Geometry: final body of the model. Coordinates: model frame, mm. A direction names the side the tool comes from. Coordinates: 2 decimals unless noted, no trailing zeros. Write each loop counter-clockwise with the first axis right and the second up, starting at its lowest first coordinate (ties: lowest second). Pieces come first, ordered by that corner, then holes. Notation, with made-up numbers: (75.25, -18) -> (80.25, -18) arc R18 ccw to (80.25, 1) -> close; hole circle Ø1 at (32.25, -15.75). An arc over 180 degrees is marked (long way). Answer as a JSON object with one key per item and string values. Group by question number.
```python
from build123d import *

# Parameters (mm, degrees)
F0_W     = 2000
F0_H     = 500
F1_DEPTH = 1000
F2_W     = 1797.4397540092
F2_H     = 308.4638491273
F3_DEPTH = 1000.001
F4_R     = 50
F5_W     = 773.9472016692
F5_H     = 195.3730471432
F6_DEPTH = 2000.001
F7_R     = 50
F8_SCALE = 0.5


with BuildPart() as f1:
    # F0 (on Front) → F1 (new body)
    with BuildSketch(Plane.XZ):
        with Locations((0, -36.5384618746)):
            Rectangle(F0_W, F0_H)
    extrude(amount=F1_DEPTH)

    # F2 (on face) → F3 (cut, through all)
    with BuildSketch(Plane.XZ.offset(1000)):
        with Locations((1.2095868587, -38.0935780704)):
            Rectangle(F2_W, F2_H)
    extrude(amount=-F3_DEPTH, mode=Mode.SUBTRACT)

    # F4
    f4_edges = [f1.edges().sort_by_distance(p)[0] for p in [
        (1000, -500, 213.461538),
        (1000, -500, -286.538462),
        (-1000, -500, 213.461538),
        (-1000, -500, -286.538462),
        (-897.51029, -500, 116.138346),
        (-897.51029, -500, -192.325503),
        (899.929464, -500, 116.138346),
        (899.929464, -500, -192.325503),
    ]]
    fillet(f4_edges, radius=F4_R)

    # F5 (on face) → F6 (cut, through all)
    with BuildSketch(Plane(origin=(-1000, 0, 0), x_dir=(0, -1, 0), z_dir=(-1, 0, 0))):
        with Locations((502.0684786141, -36.3542791456)):
            Rectangle(F5_W, F5_H)
    extrude(amount=-F6_DEPTH, mode=Mode.SUBTRACT)

    # F7
    f7_edges = [f1.edges().sort_by_distance(p)[0] for p in [
        (949.964732, -115.094878, 61.332244),
        (949.964732, -889.042079, 61.332244),
        (949.964732, -115.094878, -134.040803),
        (949.964732, -889.042079, -134.040803),
        (-948.755145, -889.042079, -134.040803),
        (-948.755145, -889.042079, 61.332244),
        (-948.755145, -115.094878, 61.332244),
        (-948.755145, -115.094878, -134.040803),
    ]]
    fillet(f7_edges, radius=F7_R)


with BuildPart() as f1_1:
    # F8: moved
    add(f1.part.scale(F8_SCALE))


solid = f1_1.part
```
Item 1: Mould query, pull axis Z, two halves, no side actions, for faces 4 (the cylindrical face through (-492.871, -253.5, 99.213)), 5 (the flat face through (-500, -246, -86)), 6 (the cylindrical face through (-474.019, -437.003, -59.891)). Classes: +Z half, -Z half, draft (parallel to the pull), parting line (faces both ways), or undercut.
Item 2: Section B-B on z = -10.5. Output: boundary loops of the cut face in (x, y), then the cut area to 3 significant figures.
Item 3: Set-up query: faces 1 (the flat face through (-7, -500, 67)), 2 (the cylindrical face through (475.33, -437.39, 23.15)), 3 (the flat face through (-448.755, -214, -69)). Return all of +Z, -Z, +X, -X, +Y, -Y with unobstructed straight access to the full face (end or side cutting, diameter ignored); none if empty.
Item 4: Section C-C on y = -223. Output: boundary loops of the cut face in (x, z).
Item 5: Ray query, L1, parallel to X at y = -406, z = -70; L2, parallel to Z at x = 404, y = -142; L3, parallel to X at y = -249.5, z = 88. Return the intervals inside material, ascending. Write a range as [from, to].
Item 6: Section A-A on x = 157.5. Output: boundary loops of the cut face in (y, z), then the cut area to 3 significant figures.
Item 7: Section D-D on z = -85. Output: boundary loops of the cut face in (x, y), then the cut area to 3 significant figures.
Answer sheet:
{
 "1": {"face 4": "+Z half", "face 5": "draft", "face 6": "undercut"},
 "2": {"outline": "(-500, -500) -> (-448.76, -500) -> (-448.76, -444.52) -> (-500, -444.52) -> close; (-500, -57.55) -> (-448.76, -57.55) -> (-448.76, 0) -> (-500, 0) -> close; (449.96, -500) -> (500, -500) -> (500, -444.52) -> (449.96, -444.52) -> close; (449.96, -57.55) -> (500, -57.55) -> (500, 0) -> (449.96, 0) -> close", "area": "11,400 mm^2"},
 "3": {"face 1": "+Z, -Z, +X, -X, -Y", "face 2": "+X, -X", "face 3": "+Y, -Y"},
 "4": {"outline": "(-500, -118.27) arc R25 ccw to (-475, -143.27) -> (475, -143.27) arc R25 ccw to (500, -118.27) -> (500, -67.02) -> (449.96, -67.02) -> (449.96, -71.16) arc R25 cw to (424.96, -96.16) -> (-423.76, -96.16) arc R25 cw to (-448.76, -71.16) -> (-448.76, -67.02) -> (-500, -67.02) -> close; (-500, 30.67) -> (-448.76, 30.67) -> (-448.76, 33.07) arc R25 cw to (-423.76, 58.07) -> (424.96, 58.07) arc R25 cw to (449.96, 33.07) -> (449.96, 30.67) -> (500, 30.67) -> (500, 81.73) arc R25 ccw to (475, 106.73) -> (-475, 106.73) arc R25 ccw to (-500, 81.73) -> close"},
 "5": {"L1": "x = [-500, -448.76], [449.96, 500]", "L2": "z = [-143.27, -96.16], [58.07, 106.73]", "L3": "x = [-499.2, 499.2]"},
 "6": {"outline": "(-500, -143.27) -> (0, -143.27) -> (0, -96.16) -> (-500, -96.16) -> close; (-500, 58.07) -> (0, 58.07) -> (0, 106.73) -> (-500, 106.73) -> close", "area": "47,900 mm^2"},
 "7": {"outline": "(-500, -500) -> (-444.58, -500) -> (-444.58, 0) -> (-500, 0) -> close; (445.79, -500) -> (500, -500) -> (500, 0) -> (445.79, 0) -> close", "area": "54,800 mm^2"}
}
